Could you check a few things on this drawing? It's one solid part, dimensions in mm from its lowest x, y, z. Round coordinates to 2 decimals unless told otherwise and drop trailing zeros. Write each loop counter-clockwise with the first axis right and the second up, starting at its lowest first coordinate (ties: lowest second). Pieces come first, ordered by that corner, then holes. Notation, with made-up numbers: (49, -22) -> (66, -22) arc R14 ccw to (66, 1) -> close; hole circle Ø9 at (24, 80). An arc over 180 degrees is marked (long way). Put each result on its own line as item: value. Start each with the question number.
1) If I drill on line 1 along Y through (x, z) = (12.5, 10); line 2 along X through (y, z) = (290, 17.75); line 3 along X through (y, z) = (108.5, 17), over which ranges is the centre line in solid material (lowest first)? Write a range as [from, to].
2) I want a section at A-A, the plane z = 16. List the corners of the cut face in (x, y) for me.
3) Will this pin go through, and if not, where does the flat tip stop? P1, Ø4, axis at y = 130, z = 10, coming from the -X side (3 decimals).
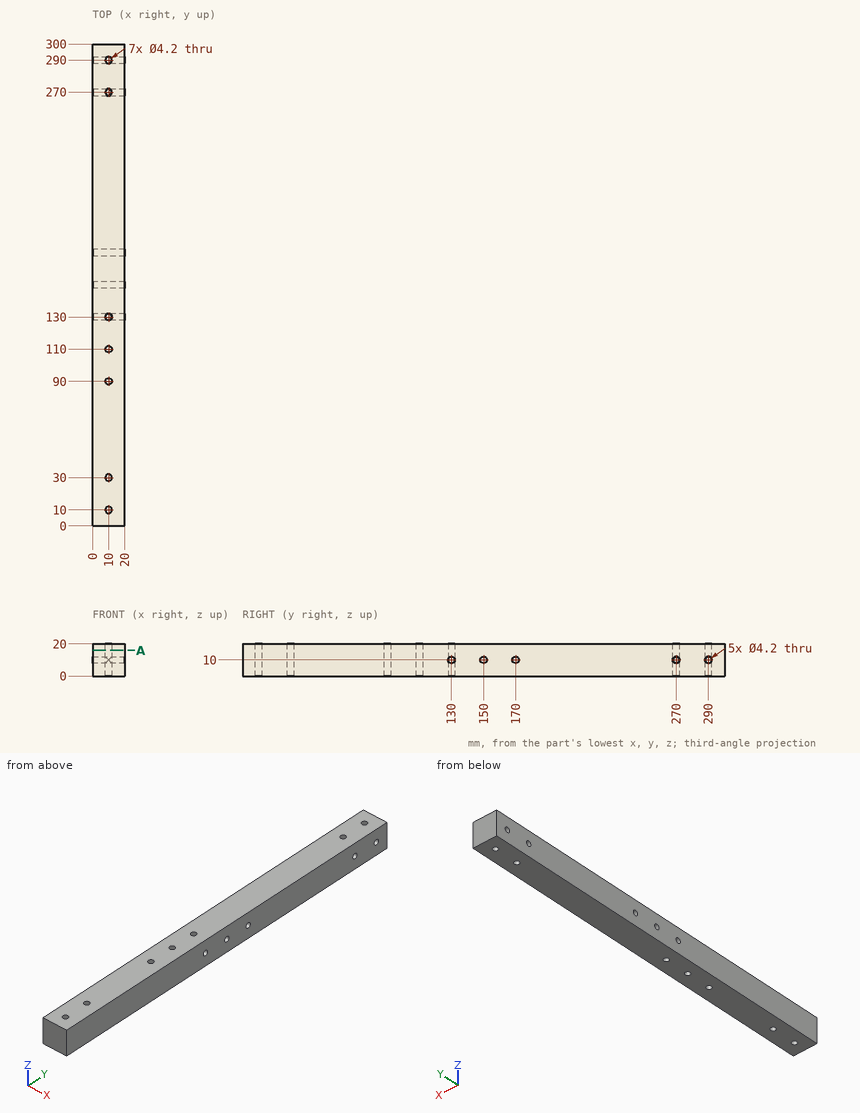
Findings:
1. line 1: y = [0, 127.9], [132.1, 147.9], [152.1, 167.9], [172.1, 267.9], [272.1, 287.9], [292.1, 300]
1. line 2: x = [0, 7.9], [12.1, 20]
1. line 3: x = [0, 8.53], [11.47, 20]
2. outline: (0, 0) -> (20, 0) -> (20, 300) -> (0, 300) -> close; hole circle Ø4.2 at (10, 10); hole circle Ø4.2 at (10, 30); hole circle Ø4.2 at (10, 90); hole circle Ø4.2 at (10, 110); hole circle Ø4.2 at (10, 130); hole circle Ø4.2 at (10, 270); hole circle Ø4.2 at (10, 290)
3. P1: passes through
